Verification items for the finished model (mm, model axes). Coordinates: 2 decimals unless noted, no trailing zeros. Loops run counter-clockwise (first coordinate to the right, second up) from the corner with the lowest first, then second, coordinate; pieces in that order, holes last. Notation, with made-up numbers: M 7.25,50 L 12.25,50 A13 ccw 12.25,68 Z; hole C -38,-17.5 d6. An arc over 180 degrees is marked long. Write item = value, one per line. Start each with the question number.
```python
from build123d import *

# Parameters (mm, degrees)
BOSS_EXTRUDE1_DEPTH             = 10
BOSS_EXTRUDE2_DEPTH             = 10
F_5_0MM_DOWEL_HOLE2_D           = 5
F_5_0MM_DOWEL_HOLE2_CSINK_D     = 5.05
F_5_0MM_DOWEL_HOLE2_CSINK_ANGLE = 90


with BuildPart() as part:
    # Sketch1 → Boss-Extrude1 (new body)
    with BuildSketch(Plane(origin=(0, 0, 0), x_dir=(1, 0, 0), z_dir=(0, 1, 0))):
        Polygon((0, 0), (101.6, 0), (126.970266889, -50.770266889), (176.970266889, -50.770266889), (136.243205185, -35.770266889), (110.872938296, 15), (0, 15), align=None)
    extrude(amount=BOSS_EXTRUDE1_DEPTH)

    # Sketch2 → Boss-Extrude2 (add)
    with BuildSketch(Plane(origin=(0, 10, 0), x_dir=(1, 0, 0), z_dir=(0, 1, 0))):
        with BuildLine():
            Line((0, 15), (0, 0))
            ThreePointArc((0, 0), (-7.5, 7.5), (0, 15))
        make_face()
    extrude(amount=-BOSS_EXTRUDE2_DEPTH)

    # Ø5.0mm Dowel Hole2 (through all)
    with Locations(Plane(origin=(0, 10, 0), x_dir=(1, 0, 0), z_dir=(0, 1, 0))):
        with Locations((0, 7.5)):
            CounterSinkHole(F_5_0MM_DOWEL_HOLE2_D / 2, F_5_0MM_DOWEL_HOLE2_CSINK_D / 2, counter_sink_angle=F_5_0MM_DOWEL_HOLE2_CSINK_ANGLE)


solid = part.part
```
Q1. Scan lines: L1, parallel to Z at x = 0, y = 7.5; L2, parallel to X at y = 5.5, z = -8.5; L3, parallel to Z at x = 43.5, y = 0.5. Record each from-to range of solid material in increasing order. Write a range as [from, to].
Q2. Sectioned sample at A-A on y = 6. Record the cut outline in (x, z).
Q3. Sectioned sample at D-D on z = 27. Record the cut outline in (x, y), plus the area to 3 significant figures.
Q4. Sectioned sample at B-B on z = -7.5. Record the cut outline in (x, y) (3 decimals).
Q5. Sectioned sample at C-C on x = 95. Record the cut outline in (y, z), plus the area to 3 significant figures.
Q6. Mould release check, pull along X, two halves, no side actions. Record for faces 1 (the face through (50, 5, 0)), 2 (the face through (114.108, 4.93, 25.03)), 3 (the face through (0.54, 4.92, -5.06)): +X half, -X half, draft (parallel to the pull), parting line (faces both ways), or undercut.
Q7. Gauge pin test, flat ends, axial feed: pin 1 (6 mm diameter, centred on y = 1.5, z = 19, fed in from +X); pin 2 (1.5 mm diameter, centred on x = 157.5, y = 7, fed in from -Z); pin 3 (6 mm diameter, centred on x = 143, y = 2.5, fed in from -Z). Record the tip position at first contact, or that the pin passes through.
Solutions:
q1.L1 = [-15, -10], [-5, 0]
q1.L2 = [-7.43, -2.29], [2.29, 114.12]
q1.L3 = [-15, 0]
q2.outline = M 0,-15 L 110.87,-15 L 136.24,35.77 L 176.97,50.77 L 126.97,50.77 L 101.6,0 L 0,0 A7.5 ccw Z; hole C 0,-7.5 d5
q3.outline = M 115.09,0 L 131.86,0 L 131.86,10 L 115.09,10 Z
q3.area = 168 mm²
q4.outline = M -7.5,0 L -2.5,0 L -2.5,9.975 L -2.525,10 L -7.5,10 Z; M 2.5,0 L 114.621,0 L 114.621,10 L 2.525,10 L 2.5,9.975 Z
q5.outline = M 0,-15 L 10,-15 L 10,0 L 0,0 Z
q5.area = 150 mm²
q6.face_1 = draft
q6.face_2 = -X half
q6.face_3 = undercut
q7.pin_1 = 129.36
q7.pin_2 = 43.32
q7.pin_3 = 37.15
